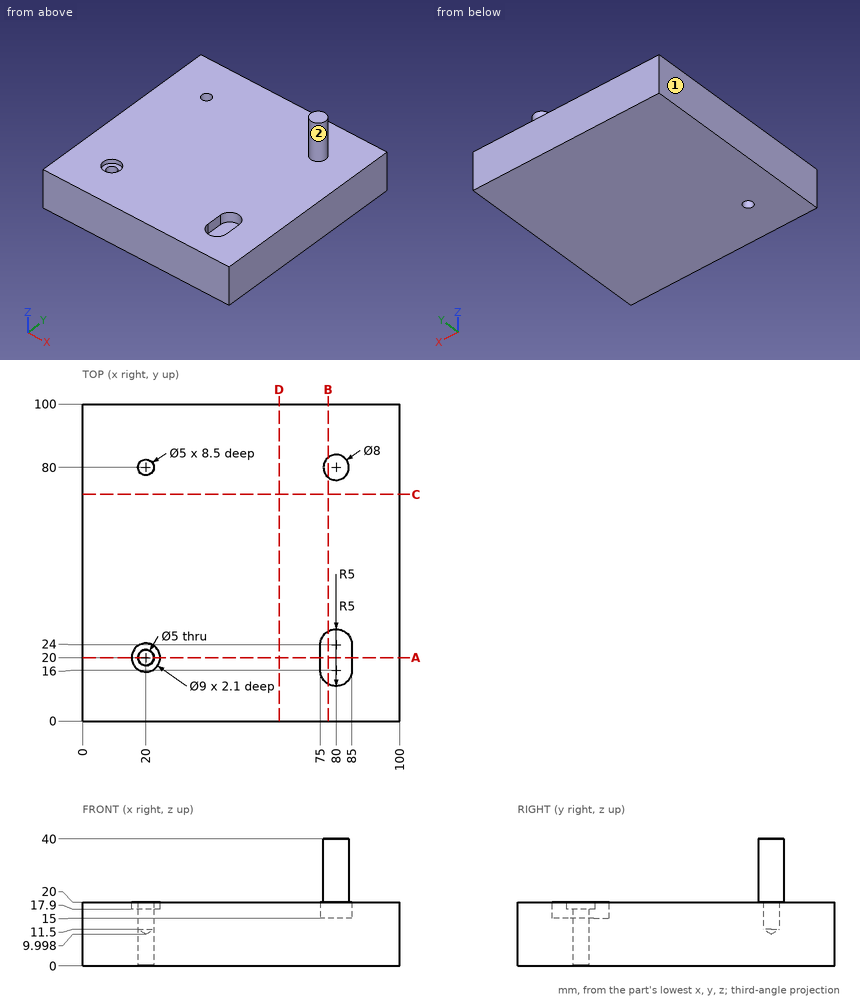
Verification items for this drawing (mm, ordinates from the low corner). A direction names the side the tool comes from. Coordinates: 2 decimals unless noted, no trailing zeros. Write each loop counter-clockwise with the first axis right and the second up, starting at its lowest first coordinate (ties: lowest second). Pieces come first, ordered by that corner, then holes. Notation, with made-up numbers: M 79.25,73.5 L 114.25,73.5 A32 cw 114.25,100.5 Z; hole C -31.5,-2 d8. An arc over 180 degrees is marked long. Answer as a JSON object with one key per item and string values.
1. Section check B-B, the plane x = 77.5. Enter the section's corners in (y, z).
Answers below:
{"outline": "M 0,0 L 100,0 L 100,20 L 83.12,20 L 83.12,40 L 76.88,40 L 76.88,20 L 28.33,20 L 28.33,15 L 11.67,15 L 11.67,20 L 0,20 Z"}
2. Scan lines: L1, parallel to Y at x = 20, z = 14.5; L2, parallel to Y at x = 20, z = 19; L3, parallel to Y at x = 20, z = 9. Record each from-to range of solid material in increasing order.
Answers below:
{"L1": "y = 0 to 17.5, 22.5 to 77.5, 82.5 to 100", "L2": "y = 0 to 15.5, 24.5 to 77.5, 82.5 to 100", "L3": "y = 0 to 17.5, 22.5 to 100"}
3. Tool access check on the marked faces 1 and 2. Record the directions out of +Z, -Z, +X, -X, +Y, -Y that give a thin tool (end or side, any length) a straight path to the whole face; none if there is none.
Answers below:
{"face 1": "+Z, -Z, -X, +Y, -Y", "face 2": "+Z"}
4. Go/stop test with flat-tipped pins: pin 1 Ø12 at (x, y) = (50, 45) entering from +Z; pin 2 Ø5 at (y, z) = (71.5, 28.5) entering from -X. Record where each tip stops, or that it passes through.
Answers below:
{"pin 1": "stops at z = 20", "pin 2": "passes through"}
5. Section check C-C, the plane y = 71.5. Enter the section's corners in (x, z).
Answers below:
{"outline": "M 0,0 L 100,0 L 100,20 L 0,20 Z"}
6. Section check A-A, the plane y = 20. Enter the section's corners in (x, z), plus the area to 3 significant figures.
Answers below:
{"outline": "M 0,0 L 17.5,0 L 17.5,17.9 L 15.5,17.9 L 15.5,20 L 0,20 Z; M 22.5,0 L 100,0 L 100,20 L 85,20 L 85,15 L 75,15 L 75,20 L 24.5,20 L 24.5,17.9 L 22.5,17.9 Z", "area": "1,840 mm²"}
